Source: CAD feature listing. Evaluate the final solid. Frame: model axes, mm. Face numbers are marked on the shaded views. A direction names the side the tool comes from. Coordinates: 2 decimals unless noted, no trailing zeros. Loops run counter-clockwise (first coordinate to the right, second up) from the corner with the lowest first, then second, coordinate; pieces in that order, holes last.
Item 1: Pin query (flat end, axial travel): pin 1 Ø12 at (y, z) = (30, 9.5) entering from -X; pin 2 Ø20 at (x, y) = (16, 33.5) entering from +Z; pin 3 Ø2 at (x, z) = (31.5, 7.5) entering from +Y; pin 4 Ø2.5 at (x, y) = (5, 55) entering from -Z. Return the tip coordinate at first contact, or that it passes through.
Item 2: Section query B-B, the plane y = 55. Return the cut outline in (x, z).
Item 3: Section query C-C, the plane x = 35. Return the cut outline in (y, z), then the cut area to 3 significant figures.
Item 4: Section query A-A, the plane z = 35. Return the cut outline in (x, y).
Item 5: Section query D-D, the plane x = 9.5. Return the cut outline in (y, z).
Item 6: Reachability of the marked faces 1 and 2 from +Z, -Z, +X, -X, +Y, -Y: full face, straight path, thin tool, end or side. Return the list, or none.
Item 7: Line query: probe 1 along Y at (x, z) = (35, 3.75); probe 2 along X at (y, z) = (15, 1.55); probe 3 along Z at (x, y) = (5, 2). Output: solid intervals per line, ascending.
```python
from build123d import *

# Parameters (mm, degrees)
F1_DEPTH = 40
F3_D     = 4.4
F5_D     = 4.4
F6_R     = 1


with BuildPart() as f1:
    # F0 (on Right) → F1 (new body)
    with BuildSketch(Plane.YZ):
        Polygon((5, 40), (0, 40), (0, 0), (60, 0), (60, 5), (5, 5), align=None)
    extrude(amount=F1_DEPTH)

    # F3 (through all)
    with Locations(Plane(origin=(0, 5, 0), x_dir=(-1, 0, 0), z_dir=(0, 1, 0))):
        with Locations((-35, 35), (-5, 35), (-5, 10), (-35, 10)):
            Hole(F3_D / 2)

    # F5 (through all)
    with Locations(Plane(origin=(0, 0, 0), x_dir=(1, 0, 0), z_dir=(0, 0, -1))):
        with Locations((35, -55), (5, -55), (5, -15), (35, -15)):
            Hole(F5_D / 2)

    # F6
    f6_edges = [f1.edges().sort_by_distance(p)[0] for p in [
        (40, 60, 2.5),
        (0, 60, 2.5),
        (20, 60, 0),
        (0, 30, 0),
        (20, 0, 0),
        (40, 30, 0),
    ]]
    fillet(f6_edges, radius=F6_R)


solid = f1.part
```
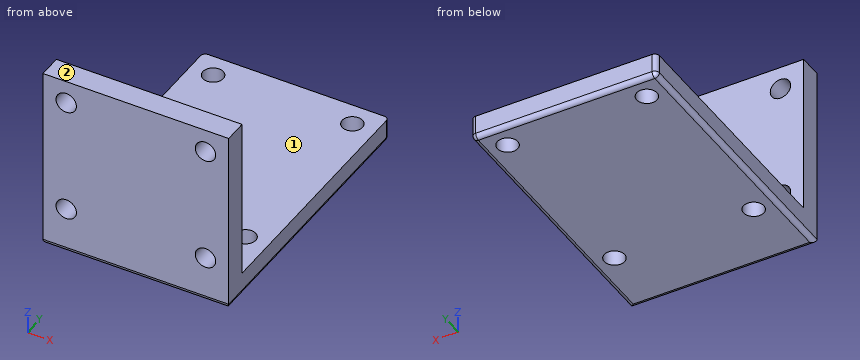
Verdict:
1. pin 1: stops at x = 0
1. pin 2: stops at z = 5
1. pin 3: stops at y = 5
1. pin 4: passes through
2. outline: (0, 1) arc R1 ccw to (1, 0) - (2.8, 0) - (2.8, 5) - (0, 5) - close; (7.2, 0) - (32.8, 0) - (32.8, 5) - (7.2, 5) - close; (37.2, 0) - (39, 0) arc R1 ccw to (40, 1) - (40, 5) - (37.2, 5) - close
3. outline: (0, 1) arc R1 ccw to (1, 0) - (12.8, 0) - (12.8, 5) - (5, 5) - (5, 7.8) - (0, 7.8) - close; (0, 12.2) - (5, 12.2) - (5, 32.8) - (0, 32.8) - close; (0, 37.2) - (5, 37.2) - (5, 40) - (0, 40) - close; (17.2, 0) - (52.8, 0) - (52.8, 5) - (17.2, 5) - close; (57.2, 0) - (59, 0) arc R1 ccw to (60, 1) - (60, 5) - (57.2, 5) - close
3. area: 387 mm2
4. outline: (0, 0) - (2.8, 0) - (2.8, 5) - (0, 5) - close; (7.2, 0) - (32.8, 0) - (32.8, 5) - (7.2, 5) - close; (37.2, 0) - (40, 0) - (40, 5) - (37.2, 5) - close
5. outline: (0, 1) arc R1 ccw to (1, 0) - (59, 0) arc R1 ccw to (60, 1) - (60, 5) - (5, 5) - (5, 40) - (0, 40) - close
6. face 1: +Z, +X, -X, +Y
6. face 2: +Z, +X, -X, +Y, -Y
7. probe 1: y = 0 to 12.8, 17.2 to 52.8, 57.2 to 60
7. probe 2: x = 0 to 2.8, 7.2 to 32.8, 37.2 to 40
7. probe 3: z = 0 to 7.8, 12.2 to 32.8, 37.2 to 40
